Work out the finished part from the listing and answer in its coordinate system (mm). A direction names the side the tool comes from. Coordinates: 2 decimals unless noted, no trailing zeros. Write each loop counter-clockwise with the first axis right and the second up, starting at its lowest first coordinate (ties: lowest second). Pieces come first, ordered by that corner, then holes. Notation, with made-up numbers: (83, 26) - (141, 26) arc R7 cw to (141, 38) - close; hole circle Ø5 at (23, -36.75). An arc over 180 degrees is marked (long way). Use one line per item in the form item = value. Start each with the question number.
Item 1: Given pin 1 (1.5 mm diameter, centred on x = 3.5, y = 5, fed in from -Z); pin 2 (1 mm diameter, centred on x = 3, y = 10, fed in from -Z); pin 3 (8 mm diameter, centred on y = 13.5, z = 1, fed in from -X); pin 4 (3 mm diameter, centred on x = -4, y = 8, fed in from +Z), each flat-ended and moving along its own axis, determine where each tip first touches the part or whether it passes through.
Item 2: For faces 4 (the cylindrical face through (-0.132, 6.087, -5.49)), 5 (the flat face through (0, 10.16, 0)), determine the directions among +Z, -Z, +X, -X, +Y, -Y from which every point of the face is accessible in a straight line to the end or side of a thin tool.
Item 3: A cutting plane is placed at D-D (z = -5.25). Write down the section's boundary in (x, y), then the cut area to 3 significant figures.
Item 4: A cutting plane is placed at B-B (z = 0). Write down the section's boundary in (x, y).
Item 5: Consider probe 1 along X at (y, z) = (12.75, 0); probe 2 along Z at (x, y) = (0, 2.75); probe 3 along Y at (x, z) = (4.75, 5.75). Determine where each line is inside the solid, lowest interval first.
Item 6: A cutting plane is placed at A-A (x = 0). Write down the section's boundary in (y, z), then the cut area to 3 significant figures.
Item 7: Determine the mould class of faces 1 (the cylindrical face through (-0.132, 6.087, 5.49)), 2 (the flat face through (5, 0, 1)), 3 (the cylindrical face through (9.135, 13.379, -0.132)) for opening direction Y: released by +Y, released by -Y, zero draft, split by the parting line, or undercut.
from build123d import *

# Parameters (mm, degrees)
SKETCH1_R                           = 6.35
BOSS_EXTRUDE1_DEPTH                 = 10.16
SKETCH2_R                           = 4.7625
CUT_EXTRUDE2_DEPTH                  = 10.16
SKETCH3_R                           = 6.35
BOSS_EXTRUDE2_DEPTH                 = 6.35
CUT_EXTRUDE3_REACH                  = 20.794
CUT_EXTRUDE3_END_RADIUS             = 6.35
SKETCH4_R                           = 1.016
CUT_EXTRUDE3_DIRECTION_2_REACH      = 20.794
CUT_EXTRUDE3_DIRECTION_2_END_RADIUS = 6.35
BOSS_EXTRUDE3_START                 = -6.35
SKETCH5_R                           = 10.16
SKETCH5_R_2                         = 6.35
BOSS_EXTRUDE3_DEPTH                 = 6.35
SKETCH10_R                          = 1.016
CUT_EXTRUDE4_DEPTH                  = 6.35


with BuildPart() as part:
    # Sketch1 → Boss-Extrude1 (new body)
    with BuildSketch(Plane(origin=(0, 0, 0), x_dir=(1, 0, 0), z_dir=(0, 1, 0))):
        with Locations(Location((0, 0, 0), (0, 0, 270))):
            Circle(SKETCH1_R)
    extrude(amount=BOSS_EXTRUDE1_DEPTH)

    # Sketch2 → Cut-Extrude2 (cut)
    with BuildSketch(Plane(origin=(0, 10.16, 0), x_dir=(1, 0, 0), z_dir=(0, 1, 0))):
        with Locations(Location((0, 0, 0), (0, 0, 270))):
            Circle(SKETCH2_R)
    extrude(amount=-CUT_EXTRUDE2_DEPTH, mode=Mode.SUBTRACT)

    # Sketch3 → Boss-Extrude2 (add)
    with BuildSketch(Plane(origin=(0, 10.16, 0), x_dir=(1, 0, 0), z_dir=(0, 1, 0))):
        with Locations(Location((0, 0, 0), (0, 0, 270))):
            Circle(SKETCH3_R)
    extrude(amount=BOSS_EXTRUDE2_DEPTH)

    # Cut-Extrude3: up to this cylinder (the profile starts inside it)
    cut_extrude3_end = Plane(origin=(0, 5.08, 0), z_dir=(0, -1, 0)) * Cylinder(CUT_EXTRUDE3_END_RADIUS, 55.288, mode=Mode.PRIVATE)
    # Sketch4 → Cut-Extrude3 (cut, up to the surface)
    with BuildSketch(Plane.XY, mode=Mode.PRIVATE) as cut_extrude3_sk1:
        with Locations((0, 5.08)):
            Circle(SKETCH4_R)
    cut_extrude3_tool1 = extrude(cut_extrude3_sk1.sketch, amount=-CUT_EXTRUDE3_REACH, mode=Mode.PRIVATE) & cut_extrude3_end
    add(cut_extrude3_tool1.solids().sort_by_distance((0, 5.08, 0))[0], mode=Mode.SUBTRACT)

    # Cut-Extrude3 direction 2: up to this cylinder (the profile starts inside it)
    cut_extrude3_direction_2_end = Plane(origin=(0, 5.08, 0), z_dir=(0, -1, 0)) * Cylinder(CUT_EXTRUDE3_DIRECTION_2_END_RADIUS, 55.288, mode=Mode.PRIVATE)
    # Sketch4 → Cut-Extrude3 direction 2 (cut, up to the surface)
    with BuildSketch(Plane.XY, mode=Mode.PRIVATE) as cut_extrude3_direction_2_sk1:
        with Locations((0, 5.08)):
            Circle(SKETCH4_R)
    cut_extrude3_direction_2_tool1 = extrude(cut_extrude3_direction_2_sk1.sketch, amount=CUT_EXTRUDE3_DIRECTION_2_REACH, mode=Mode.PRIVATE) & cut_extrude3_direction_2_end
    add(cut_extrude3_direction_2_tool1.solids().sort_by_distance((0, 5.08, 0))[0], mode=Mode.SUBTRACT)

    # Sketch5 → Boss-Extrude3 (add)
    with BuildSketch(Plane(origin=(0, 16.51, 0), x_dir=(1, 0, 0), z_dir=(0, 1, 0)).offset(BOSS_EXTRUDE3_START)):
        with Locations(Location((0, 0, 0), (0, 0, 270))):
            Circle(SKETCH5_R)
        with Locations(Location((0, 0, 0), (0, 0, 270))):
            Circle(SKETCH5_R_2, mode=Mode.SUBTRACT)
    extrude(amount=BOSS_EXTRUDE3_DEPTH)

    # Sketch10 → Cut-Extrude4 (cut)
    with BuildSketch(Plane(origin=(0, 16.51, 0), x_dir=(1, 0, 0), z_dir=(0, 1, 0))):
        with Locations(Location((8.128, 0, 0), (0, 0, 270))):
            Circle(SKETCH10_R)
        with Locations(Location((-8.128, 0, 0), (0, 0, 270))):
            Circle(SKETCH10_R)
    extrude(amount=-CUT_EXTRUDE4_DEPTH, mode=Mode.SUBTRACT)


solid = part.part
Answer:
q1.pin_1 = -5.72
q1.pin_2 = -9.84
q1.pin_3 = -10.16
q1.pin_4 = 5.84
q2.face_4 = +Z, -Z
q2.face_5 = -Y
q3.outline = (-8.7, 10.16) - (-3.57, 10.16) - (-3.57, 0) - (3.57, 0) - (3.57, 10.16) - (8.7, 10.16) - (8.7, 16.51) - (-8.7, 16.51) - close; hole circle Ø2.03 at (0, 5.08)
q3.area = 180 mm²
q4.outline = (-10.16, 10.16) - (-9.14, 10.16) - (-9.14, 16.51) - (-10.16, 16.51) - close; (-7.11, 10.16) - (-6.35, 10.16) - (-6.35, 0) - (-4.76, 0) - (-4.76, 10.16) - (4.76, 10.16) - (4.76, 0) - (6.35, 0) - (6.35, 10.16) - (7.11, 10.16) - (7.11, 16.51) - (-7.11, 16.51) - close; (9.14, 10.16) - (10.16, 10.16) - (10.16, 16.51) - (9.14, 16.51) - close
q5.probe_1 = -10.16 to -9.14, -7.11 to 7.11, 9.14 to 10.16
q5.probe_2 = -6.35 to -4.76, 4.76 to 6.35
q5.probe_3 = 10.16 to 16.51
q6.outline = (0, -6.35) - (4.06, -6.35) - (4.06, -4.76) - (0, -4.76) - close; (0, 4.76) - (4.06, 4.76) - (4.06, 6.35) - (0, 6.35) - close; (6.1, -6.35) - (10.16, -6.35) - (10.16, -10.16) - (16.51, -10.16) - (16.51, 10.16) - (10.16, 10.16) - (10.16, 6.35) - (6.1, 6.35) - (6.1, 4.76) - (10.16, 4.76) - (10.16, -4.76) - (6.1, -4.76) - close
q6.area = 155 mm²
q7.face_1 = undercut
q7.face_2 = released by -Y
q7.face_3 = zero draft
